from build123d import *

# Parameters (mm, degrees)
F1_DEPTH     = 55
F1_TAPER     = -15
F4_DEPTH     = 55
F4_TAPER     = -12
F5_W         = 5
F5_H         = 130
F6_DEPTH     = 47
F10_W        = 360.01701653
F10_H        = 225.87454319
F11_DEPTH    = 25
F12_W        = 5
F12_H        = 46
F13_DEPTH    = 15
F14_W        = 5
F14_H        = 46
F15_DEPTH    = 15
F8_W         = 54.0339685977
F8_H         = 90.1
F16_DEPTH    = 32.6
F9_W         = 55.9400806222
F9_H         = 89.7377200425
F17_DEPTH    = 25
F18_W        = 347.7291613817
F18_H        = 217.2330617905
F19_DEPTH    = 25
F20_W        = 34.4053636551
F20_H        = 45.9854951713
F21_DEPTH    = 25
F22_W        = 1.5565819549
F22_H        = 85.7377200425
F22_W_2      = 27.4434180451
F23_DEPTH    = 52
F24_T1_DEPTH = 114.7377200425
F26_DEPTH    = 25
F27_W        = 5
F27_H        = 32
F28_DEPTH    = 10
F29_W        = 5
F29_H        = 35
F30_DEPTH    = 8
F31_W        = 122.5292943418
F31_H        = 48.8124843687
F32_DEPTH    = 25
F33_W        = 5
F33_H        = 6
F33_W_2      = 6
F34_DEPTH    = 32


# Not quite as in the source:
# - a fillet or chamfer that OpenCascade refuses, or shapes differently, is made with other operations: its cross-section is extruded or revolved along the edge and cut away or added
# - ends of sketch curves that miss each other by under 0.0002 mm in the source are joined


with BuildPart() as f1:
    # F0 (on Front) → F1 (new body)
    with BuildSketch(Plane.XZ):
        with BuildLine():
            Line((34.0782237053, 85.1892769337), (-105.9217762947, 85.1892769337))
            ThreePointArc((-105.9217762947, 85.1892769337), (-120.0639119184, 79.3314125574), (-125.9217762947, 65.1892769337))
            Line((-125.9217762947, 65.1892769337), (-125.9217762947, -24.8107230663))
            ThreePointArc((-125.9217762947, -24.8107230663), (-120.0639119184, -38.9528586901), (-105.9217762947, -44.8107230663))
            Line((-105.9217762947, -44.8107230663), (34.0782237053, -44.8107230663))
            ThreePointArc((34.0782237053, -44.8107230663), (48.220359329, -38.9528586901), (54.0782237053, -24.8107230663))
            Line((54.0782237053, -24.8107230663), (54.0782237053, 65.1892769337))
            ThreePointArc((54.0782237053, 65.1892769337), (48.220359329, 79.3314125574), (34.0782237053, 85.1892769337))
        make_face()
    extrude(amount=F1_DEPTH, taper=F1_TAPER)

    # F3 (on offset) → F4 (cut)
    with BuildSketch(Plane.XZ.offset(5)):
        with BuildLine():
            Line((34.106137666, 85.2195297501), (-105.893862334, 85.2195297501))
            ThreePointArc((-105.893862334, 85.2195297501), (-120.0359979577, 79.3616653739), (-125.893862334, 65.2195297501))
            Line((-125.893862334, 65.2195297501), (-125.893862334, -24.7804702499))
            ThreePointArc((-125.893862334, -24.7804702499), (-120.0359979577, -38.9226058736), (-105.893862334, -44.7804702499))
            Line((-105.893862334, -44.7804702499), (34.106137666, -44.7804702499))
            ThreePointArc((34.106137666, -44.7804702499), (48.2482732898, -38.9226058736), (54.106137666, -24.7804702499))
            Line((54.106137666, -24.7804702499), (54.106137666, 65.2195297501))
            ThreePointArc((54.106137666, 65.2195297501), (48.2482732898, 79.3616653739), (34.106137666, 85.2195297501))
        make_face()
    extrude(amount=F4_DEPTH, taper=F4_TAPER, mode=Mode.SUBTRACT)

    # F5 (on face) → F6 (join)
    with BuildSketch(Plane.XZ.offset(5)):
        with Locations((-35.893862334, 20.2195297501)):
            Rectangle(F5_W, F5_H)
    extrude(amount=F6_DEPTH)

    # F10 (on Front) → F11 (cut)
    with BuildSketch(Plane.XZ):
        with Locations((5.3876563907, 10.9746605158)):
            Rectangle(F10_W, F10_H)
    extrude(amount=-F11_DEPTH, mode=Mode.SUBTRACT)

    # F12 (on face) → F13 (join)
    with BuildSketch(Plane(origin=(0, 8.8907927165, -41.8278911112), x_dir=(1, 0, 0), z_dir=(0, -0.2079116908, 0.9781476007))):
        with Locations((-35.893862334, -37.2011212889)):
            Rectangle(F12_W, F12_H)
    extrude(amount=F13_DEPTH)

    # F14 (on face) → F15 (join)
    with BuildSketch(Plane(origin=(0, 17.1148163716, 80.5188804202), x_dir=(1, 0, 0), z_dir=(0, -0.2079116908, -0.9781476007))):
        with Locations((-35.893862334, 45.6088745247)):
            Rectangle(F14_W, F14_H)
    extrude(amount=F15_DEPTH)

    # F8 (on offset) → F16 (join)
    with BuildSketch(Plane.YZ.offset(98)):
        with Locations((-27.0169842988, 19.8769969761)):
            Rectangle(F8_W, F8_H)
    extrude(amount=-F16_DEPTH)

    # F9 (on face) → F17 (join)
    with BuildSketch(Plane(origin=(50.4556696128, 13.5195559263, 0), x_dir=(-0.2588190451, 0.9659258263, 0), z_dir=(0.9659258263, 0.2588190451, 0))):
        with Locations((-41.9665145313, 20.0581369549)):
            Rectangle(F9_W, F9_H)
    extrude(amount=F17_DEPTH)

    # F18 (on Front) → F19 (cut)
    with BuildSketch(Plane.XZ):
        with Locations((0.111065805, 20.1892703772)):
            Rectangle(F18_W, F18_H)
    extrude(amount=-F19_DEPTH, mode=Mode.SUBTRACT)

    # F20 (on face) → F21 (cut)
    with BuildSketch(Plane(origin=(0, 0, -24.8107230663), x_dir=(1, 0, 0), z_dir=(0, 0, -1))):
        Polygon((68.0166854944, 55.7510983837), (65.4, 45.9854951713), (99.8053636551, 45.9854951713), (100.283839941, 55.7510983837), align=None)
        with Locations((82.6026818275, 22.9927475857)):
            Rectangle(F20_W, F20_H)
    extrude(amount=F21_DEPTH, mode=Mode.SUBTRACT)

    # F22 (on face) → F23 (cut)
    with BuildSketch(Plane.XZ.offset(54.0339685977)):
        with Locations((67.7782909774, 20.0581369549)):
            Rectangle(F22_W, F22_H)
        with Locations((82.2782909774, 20.0581369549)):
            Rectangle(F22_W_2, F22_H)
    extrude(amount=-F23_DEPTH, mode=Mode.SUBTRACT)

    # F24: fillet of radius 5 on 2 edges, made by hand

    # F24_s2 → F24_t1 (cut)
    with BuildSketch(Plane.XY.offset(-37.3107230663)):
        with BuildLine():
            ThreePointArc((98, -49.0339685977), (96.5355339059, -52.5695025036), (93, -54.0339685977))
            Line((93, -54.0339685977), (98, -54.0339685977))
            Line((98, -54.0339685977), (98, -49.0339685977))
        make_face()
        with BuildLine():
            ThreePointArc((93, 0), (96.5355339059, -1.4644660941), (98, -5))
            Line((98, -5), (98, 0))
            Line((98, 0), (93, 0))
        make_face()
    extrude(amount=F24_T1_DEPTH, mode=Mode.SUBTRACT)

    # F25 (on face) → F26 (cut)
    with BuildSketch(Plane.XZ.offset(52)):
        Polygon((-33.3938625455, 92.2565162182), (-38.3938625455, 92.2565162182), (-38.3938625455, -53.0670173466), (-33.393862334, -53.0670173466), align=None)
    extrude(amount=F26_DEPTH, mode=Mode.SUBTRACT)

    # F27 (on face) → F28 (cut)
    with BuildSketch(Plane(origin=(0, 0, 0), x_dir=(-1, 0, 0), z_dir=(0, 1, 0))):
        with Locations((-90.5, 45.9269969761)):
            Rectangle(F27_W, F27_H)
    extrude(amount=-F28_DEPTH, mode=Mode.SUBTRACT)

    # F29 (on face) → F30 (join)
    with BuildSketch(Plane(origin=(0, 11.2026807666, -41.8089738019), x_dir=(1, 0, 0), z_dir=(0, 0.2588190451, -0.9659258263))):
        with Locations((-63.4217762947, 29.0978685544)):
            Rectangle(F29_W, F29_H)
        with Locations((-8.4217762947, 29.0978685544)):
            Rectangle(F29_W, F29_H)
    extrude(amount=F30_DEPTH)

    # F31 (on face) → F32 (cut)
    with BuildSketch(Plane(origin=(0, 0, 0), x_dir=(-1, 0, 0), z_dir=(0, 1, 0))):
        with Locations((32.052250579, -48.6711980775)):
            Rectangle(F31_W, F31_H)
    extrude(amount=F32_DEPTH, mode=Mode.SUBTRACT)

    # F33 (on face) → F34 (cut)
    with BuildSketch(Plane(origin=(0, -45.0100846867, -12.0604158431), x_dir=(1, 0, 0), z_dir=(0, -0.9659258263, -0.2588190451))):
        with Locations((-63.4217762947, -46.2838347045)):
            Rectangle(F33_W, F33_H)
        with Locations((-8.7768949285, -46.2838347045)):
            Rectangle(F33_W_2, F33_H)
    extrude(amount=-F34_DEPTH, mode=Mode.SUBTRACT)


solid = f1.part
Check sheet for the modelled part. Datum: model origin and axes. Units: mm. A direction names the side the tool comes from. Round coordinates to 2 decimals unless told otherwise and drop trailing zeros. Answer as CSV lines item,"result". Start each with the question number.
1) Section check A-A on y = -9.5. State how many separate pieces and enclosed holes the cut face has, and give its area (4 significant figures).
2) Material ranges on line 1 (X direction, y = -26, z = 67.5); line 2 (X direction, y = -21, z = 0.5); line 3 (Z direction, x = 70.5, y = -16), recorded low to high. Write a range as from..to.
3) Tool access check on faces 1 (the flat face through (-36, -52, 21)), 2 (the flat face through (-63.457, -17.016, -55.582)), 3 (the flat face through (-5.922, -14, -55)), 4 (the flat face through (67, -28, 19)), 5 (the flat face through (-10.922, -14, -55)). Record the directions out of +Z, -Z, +X, -X, +Y, -Y that give a thin tool (end or side, any length) a straight path to the whole face; none if there is none.
4) Release check for a two-part mould opening along Z. For faces 6 (the flat face through (81, -2.034, 21)), 7 (the flat face through (81, -28, -24.811)), 8 (the flat face through (-8.457, -18.569, -49.786)), 9 (the flat face through (81, -27, 64.927)) record: pulls with the +Z half, pulls with the -Z half, needs draft (parallel to the pull), parting line crosses it, or undercut.
5) Go/stop test with flat-tipped pins: P1, Ø10, axis at x = -112, y = -14, coming from the -Z side; P2, Ø8.5, axis at y = -21, z = -51.5, coming from the -X side; P3, Ø2, axis at x = -114.5, y = -11, coming from the -Z side. Record where each tip stops, or that it passes through.
Found:
1,separate pieces,"3"
1,enclosed holes,"3"
1,area,"2,855 mm^2"
2,line 1,"x = -132.79..-130.25, -38.39..-33.39, 58.46..60.95"
2,line 2,"x = -131.55..-129.29, -38.39..-33.39, 57.51..67, 96..98"
2,line 3,"z = -24.81..-22.81, 62.93..64.93"
3,face 1,"-Y"
3,face 2,"+X, -X"
3,face 3,"-Z, +X, +Y"
3,face 4,"none"
3,face 5,"-Z, +Y"
4,face 6,"undercut"
4,face 7,"pulls with the -Z half"
4,face 8,"undercut"
4,face 9,"pulls with the +Z half"
5,P1,"stops at z = -49.46"
5,P2,"stops at x = -118.65"
5,P3,"stops at z = -46.57"
